Part model, mm, in its own coordinate system. Round coordinates to 2 decimals unless told otherwise and drop trailing zeros. Write each loop counter-clockwise with the first axis right and the second up, starting at its lowest first coordinate (ties: lowest second). Pieces come first, ordered by that corner, then holes.
1) Drill centre lines: L1, parallel to X at y = 0.5, z = 1; L2, parallel to X at y = 0.95, z = 13.5. Where is each one in solid material? Low to high.
2) Pull direction X, two halves, no side cores. Call faces 1 (the flat face through (120, 2, -43)), 2 (the flat face through (-3, 2, -8)): +X half, -X half, draft (parallel to the pull), parting line (faces both ways), or undercut.
3) Saw through at A-A on z = -101.5. Write the cut outline in (x, y), and give its area (3 significant figures).
4) Saw through at B-B on x = 106.5. Write the cut outline in (y, z).
```python
from build123d import *

# Parameters (mm, degrees)
SKETCH_2_W                 = 130
SKETCH_2_H                 = 108
EXTRUDE_1_DEPTH            = 3
SKETCH_3_W                 = 5
SKETCH_3_H                 = 3
SKETCH_3_W_2               = 3
SKETCH_3_H_2               = 5
CUT_EXTRUDE_1_DEPTH        = 155.961285488
MIRROR_2_COPY_1_SKETCH_W   = 5
MIRROR_2_COPY_1_SKETCH_H   = 3
MIRROR_2_COPY_1_SKETCH_W_2 = 3
MIRROR_2_COPY_1_SKETCH_H_2 = 5
MIRROR_2_COPY_1_DEPTH      = 155.961285488
SKETCH_5_W                 = 130
SKETCH_5_H                 = 8.5
EXTRUDE_2_DEPTH            = 3
SKETCH_6_R                 = 1.6
CUT_EXTRUDE_2_DEPTH        = 161.471960168


with BuildPart() as part:
    # 草图2 → 凸台-拉伸1 (new body)
    with BuildSketch(Plane(origin=(0, 0, 0), x_dir=(1, 0, 0), z_dir=(0, 1, 0))):
        with Locations((55, 44)):
            Rectangle(SKETCH_2_W, SKETCH_2_H)
    extrude(amount=EXTRUDE_1_DEPTH)

    # 草图3 → 切除-拉伸1 (cut, through all)
    with BuildSketch(Plane(origin=(0, 3, 0), x_dir=(1, 0, 0), z_dir=(0, 1, 0))):
        with Locations((4.5, 89.5)):
            Rectangle(SKETCH_3_W, SKETCH_3_H)
        with Locations((-1.5, 80.5)):
            Rectangle(SKETCH_3_W_2, SKETCH_3_H_2)
    cut_extrude_1 = extrude(amount=-CUT_EXTRUDE_1_DEPTH, mode=Mode.SUBTRACT)

    # 镜向1: 切除-拉伸1 across plane
    add(cut_extrude_1.mirror(Plane.ZY.offset(-55)), mode=Mode.SUBTRACT)

    # 镜向2: 切除-拉伸1 across plane
    add(cut_extrude_1.mirror(Plane(origin=(0, 0, -44), x_dir=(1, 0, 0), z_dir=(0, 0, -1))), mode=Mode.SUBTRACT)

    # 镜向2 copy 1 sketch → 镜向2 copy 1 (cut, through all)
    with BuildSketch(Plane(origin=(110, 3, -88), x_dir=(-1, 0, 0), z_dir=(0, 1, 0))):
        with Locations((4.5, 89.5)):
            Rectangle(MIRROR_2_COPY_1_SKETCH_W, MIRROR_2_COPY_1_SKETCH_H)
        with Locations((-1.5, 80.5)):
            Rectangle(MIRROR_2_COPY_1_SKETCH_W_2, MIRROR_2_COPY_1_SKETCH_H_2)
    extrude(amount=-MIRROR_2_COPY_1_DEPTH, mode=Mode.SUBTRACT)

    # 草图5 → 凸台-拉伸2 (add)
    with BuildSketch(Plane(origin=(0, 3, 0), x_dir=(1, 0, 0), z_dir=(0, 1, 0))):
        with Locations((55, 102.25)):
            Rectangle(SKETCH_5_W, SKETCH_5_H)
        with Locations((55, -14.25)):
            Rectangle(SKETCH_5_W, SKETCH_5_H)
    extrude(amount=-EXTRUDE_2_DEPTH)

    # 草图6 → 切除-拉伸2 (cut, through all)
    with BuildSketch(Plane(origin=(0, 3, 0), x_dir=(1, 0, 0), z_dir=(0, 1, 0))):
        with Locations(Location((0, 101.5, 0), (0, 0, 270))):
            Circle(SKETCH_6_R)
        with Locations(Location((0, -13.5, 0), (0, 0, 270))):
            Circle(SKETCH_6_R)
        with Locations(Location((110, 101.5, 0), (0, 0, 270))):
            Circle(SKETCH_6_R)
        with Locations(Location((110, -13.5, 0), (0, 0, 270))):
            Circle(SKETCH_6_R)
    extrude(amount=-CUT_EXTRUDE_2_DEPTH, mode=Mode.SUBTRACT)


solid = part.part
```
Completed:
1. L1: x = -10 to 2, 7 to 103, 108 to 120
1. L2: x = -10 to -1.6, 1.6 to 108.4, 111.6 to 120
2. face 1: +X half
2. face 2: undercut
3. outline: (-10, 0) - (-1.6, 0) - (-1.6, 3) - (-10, 3) - close; (1.6, 0) - (108.4, 0) - (108.4, 3) - (1.6, 3) - close; (111.6, 0) - (120, 0) - (120, 3) - (111.6, 3) - close
3. area: 371 mm2
4. outline: (0, -106.5) - (3, -106.5) - (3, -91) - (0, -91) - close; (0, -88) - (3, -88) - (3, 0) - (0, 0) - close; (0, 3) - (3, 3) - (3, 18.5) - (0, 18.5) - close
